Autodesk Inventor part; units mm, degrees
ref_plane "YZ Plane" through (0, 0, 0) normal (1, 0, 0) x (0, 1, 0)
ref_plane "XZ Plane" through (0, 0, 0) normal (0, 1, 0) x (-1, 0, 0)
ref_plane "XY Plane" through (0, 0, 0) normal (0, 0, 1) x (1, 0, 0)
sketch "Sketch1" plane through (0, 0, 0) normal (1, 0, 0) x (0, 1, 0)
  circle A0 centre (0, 0) radius 25.4
  dimension "d0" = 50.8
extrude "Extrusion1" add sketch "Sketch1" along normal blind 12.7
sketch "Sketch10" plane through (12.7, 0, 0) normal (1, 0, 0) x (0, 0, -1)
  point P0 (0, 0)
  point P1 (0, 0)
hole "Hole4" at (12.7, 0, 0) direction (-1, 0, 0) diameter 18.2563 depth 2.54
sketch "Sketch11" plane through (10.16, 0, 0) normal (1, 0, 0) x (0, 0, -1)
  point P0 (0, 0)
  point P1 (0, 0)
hole "Hole7" at (10.16, 0, 0) direction (-1, 0, 0) diameter 13.0969 depth 4.7625
sketch "Sketch12" plane through (0, 0, 0) normal (-1, 0, 0) x (0, 0, 1)
  line L0 (-10.795, 15.24) -> (10.795, 15.24) construction
  line L1 (10.795, 15.24) -> (10.795, -15.24) construction
  line L2 (10.795, -15.24) -> (-10.795, -15.24) construction
  line L3 (-10.795, -15.24) -> (-10.795, 15.24) construction
  line L4 (-10.795, 15.24) -> (10.795, -15.24) construction
  line L5 (10.795, 15.24) -> (-10.795, -15.24) construction
  point P0 (0, 0)
  dimension "d107" = 21.59
  dimension "d108" = 30.48
hole "Hole8" at (0, 15.24, 10.795) at (0, -15.24, 10.795) at (0, -15.24, -10.795) at (0, 15.24, -10.795) direction (1, 0, 0) diameter 2.9464 end through all
sketch "Sketch13" plane through (0, 0, 0) normal (-1, 0, 0) x (0, 0, 1)
  point P0 (0, 0)
  point P1 (0, 0)
hole "Hole9" at (0, 0, 0) direction (1, 0, 0) diameter 1 end through all
sketch "Sketch9" plane through (0, 0, 0) normal (0, 1, 0) x (-1, 0, 0)
  line L0 (-11.4554, -11.1252) -> (-12.7, -11.1252)
  line L1 (-12.7, -11.1252) -> (-12.7, -13.6652)
  line L2 (-12.7, -13.6652) -> (-11.4554, -13.6652)
  line L3 (-11.4554, -13.6652) -> (-11.4554, -11.1252)
  line L4 (2.54, 0) -> (-15.24, 0)
  line L5 (-12.7, 25.4) -> (-12.7, -25.4)
  point P0 (0, 0)
  dimension "d55" = 2.54
  dimension "d56" = 1.2446
  dimension "d59" = 11.1252
revolve "Revolution1" cut sketch "Sketch9" angle 360 about axis through (-10, 0, 0) along (1, 0, 0)
sketch "Sketch14" plane through (0, 0, 0) normal (-1, 0, 0) x (0, 0, 1)
  line L0 (-9.5, 0) -> (9.5, 0)
  circle A0 centre (0, 0) radius 0.5
  dimension "d123" = 19
  dimension "d124" = 9.5
hole "Hole10" at (0, 0, 9.5) at (0, 0, -9.5) direction (1, 0, 0) diameter 2.159 depth 8.8646 tip angle 118
equation "\"d0\" = sensorHolderDiameter"
equation "\"d1\" = sensorHolderThickness"
equation "\"d100\" = glassTubeDiameter + 2 * glassTubeClearance"
equation "\"d107\" = shortHoleSpacing"
equation "\"d108\" = longHoleSpacing"
equation "\"d116\" = fiberDiameter + 2 * fiberClearance"
equation "\"d55\" = oRingGrooveWidth"
equation "\"d56\" = oRingGrooveDepth"
equation "\"d59\" = 0.5 * oRingID"
equation "\"d123\" = sensorBoardHoleSpacing"
equation "\"d124\" = 0.5 * d123"
equation "\"tubeHeight\" = 50.8"
equation "\"tubeWidth\" = 152.4"
equation "\"tubeLength\" = 304.8"
equation "\"tubeWallThickness\" = 3.175"
equation "\"plateOverhang\" = 6.35"
equation "\"moatWidth\" = 3.175"
equation "\"moatDepth\" = 3.175"
equation "\"tubePlateClearance\" = 0.127"
equation "\"blankCapThickness\" = 9.525"
equation "\"sensorCapThickness\" = 12.7"
equation "\"glassTubeDiameter\" = 12.7"
equation "\"glassTubeClearance\" = 0.19844"
equation "\"longHoleSpacing\" = 30.48"
equation "\"shortHoleSpacing\" = 21.59"
equation "\"sensorHolderDiameter\" = 50.8"
equation "\"sensorHolderThickness\" = 12.7"
equation "\"fiberClearence\" = 0"
equation "\"fiberDiameter\" = 1"
equation "\"fiberClearance\" = 0"
equation "\"oRingGrooveDepth\" = 1.2446"
equation "\"oRingGrooveWidth\" = 2.54"
equation "\"oRingID\" = 22.2504"
equation "\"glassTubeLength\" = 279.4"
equation "\"glassTubeID\" = 7.874"
equation "\"sensorBoardHoleSpacing\" = 19"
properties part number ".5 in hole" material "Aluminum 6061"
Here's how the part is built. I have some questions about the finished solid (model axes, mm). A direction names the side the tool comes from. Give positions to 0.01 mm unless a question says otherwise; leave off trailing zeros. Loops run counter-clockwise (first coordinate to the right, second up) from the corner with the lowest first, then second, coordinate; pieces in that order, holes last. Notation, with made-up numbers: (59, -6.75) -> (79, -6.75) arc R10 cw to (79, 3.25) -> close; hole circle Ø3 at (70, 25). An arc over 180 degrees is marked (long way). Answer as a JSON object with one key per item and string values. Group by question number.
Item 1: On a 3-axis mill with a long thin cutter (end or side, diameter ignored), from which of +Z, -Z, +X, -X, +Y, -Y can I reach the whole of each face in a straight line? I mean faces 1 (the flat face through (12.7, 11, -11)), 2 (the cylindrical face through (4.49, -0.05, -10.58)), 3 (the cylindrical face through (11.412, 5.554, 7.244)). Say none if no direction works.
Item 2: Imagine slicing it at D-D on z = 4. Write out the boundary of the cut face in (x, y), then the cut area to 3 significant figures.
Item 3: Will these pins go through, and if not, where does the flat tip stop? pin 1 (5 mm diameter, centred on x = 3, z = -9, fed in from +Y); pin 2 (2.5 mm diameter, centred on y = 15.24, z = 10.795, fed in from +X); pin 3 (1 mm diameter, centred on x = 4.5, y = -18.5, fed in from +Z); pin 4 (13.5 mm diameter, centred on y = -1, z = -0.5, fed in from +X).
Item 4: Imagine slicing it at B-B on y = -15.24. Write out the boundary of the cut face in (x, z), then the cut area to 3 significant figures.
Item 5: I need wall thicknesses on L1, parallel to Z at x = 7, y = 0; L2, parallel to Y at x = 5.75, z = -9.5; L3, parallel to Z at x = 5, y = 0. Which ranges of each line are inside material? Lowest first, please.
Item 6: Imagine slicing it at C-C on y = -3. Write out the boundary of the cut face in (x, z).
Item 7: Imagine slicing it at A-A on x = 4.5. Write out the boundary of the cut face in (y, z) (1 decimal), then the cut area to 3 significant figures.
Answer list:
{
 "1": {"face 1": "+Z, -Z, +X, +Y, -Y", "face 2": "-X", "face 3": "+X"},
 "2": {"outline": "(0, -25.08) -> (12.7, -25.08) -> (12.7, -13.07) -> (11.46, -13.07) -> (11.46, -10.38) -> (12.7, -10.38) -> (12.7, -8.21) -> (10.16, -8.21) -> (10.16, -5.18) -> (5.4, -5.18) -> (5.4, 5.18) -> (10.16, 5.18) -> (10.16, 8.21) -> (12.7, 8.21) -> (12.7, 10.38) -> (11.46, 10.38) -> (11.46, 13.07) -> (12.7, 13.07) -> (12.7, 25.08) -> (0, 25.08) -> close", "area": "539 mm2"},
 "3": {"pin 1": "stops at y = 24.55", "pin 2": "passes through", "pin 3": "stops at z = 17.92", "pin 4": "stops at x = 10.16"},
 "4": {"outline": "(0, -20.32) -> (12.7, -20.32) -> (12.7, -12.27) -> (0, -12.27) -> close; (0, -9.32) -> (12.7, -9.32) -> (12.7, 9.32) -> (0, 9.32) -> close; (0, 12.27) -> (12.7, 12.27) -> (12.7, 20.32) -> (0, 20.32) -> close", "area": "441 mm2"},
 "5": {"L1": "z = -25.4 to -10.58, -8.42 to -6.55, 6.55 to 8.42, 10.58 to 25.4", "L2": "y = -23.56 to -15.94, -14.54 to -1.08, 1.08 to 14.54, 15.94 to 23.56", "L3": "z = -25.4 to -10.58, -8.42 to -0.5, 0.5 to 8.42, 10.58 to 25.4"},
 "6": {"outline": "(0, -25.22) -> (12.7, -25.22) -> (12.7, -13.33) -> (11.46, -13.33) -> (11.46, -10.71) -> (12.7, -10.71) -> (12.7, -8.62) -> (10.16, -8.62) -> (10.16, -5.82) -> (5.4, -5.82) -> (5.4, 5.82) -> (10.16, 5.82) -> (10.16, 8.62) -> (12.7, 8.62) -> (12.7, 10.71) -> (11.46, 10.71) -> (11.46, 13.33) -> (12.7, 13.33) -> (12.7, 25.22) -> (0, 25.22) -> close"},
 "7": {"outline": "circle Ø50.8 at (0, 0); hole circle Ø2.9 at (-15.2, -10.8); hole circle Ø2.9 at (-15.2, 10.8); hole circle Ø2.2 at (0, -9.5); hole circle Ø2.2 at (0, 9.5); hole circle Ø1 at (0, 0); hole circle Ø2.9 at (15.2, -10.8); hole circle Ø2.9 at (15.2, 10.8)", "area": "1,990 mm2"}
}
